```python
from build123d import *

# Parameters (mm, degrees)
SKETCH_W        = 196
SKETCH_H        = 200
PAD_DEPTH       = 3
SKETCH001_R     = 39.5
POCKET_DEPTH    = 5
SKETCH002_R     = 3.5
POCKET001_DEPTH = 5
SKETCH003_W     = 8
SKETCH003_H     = 180
PAD001_DEPTH    = 4
SKETCH004_W     = 160
SKETCH004_H     = 8
PAD002_DEPTH    = 4


with BuildPart() as part:
    # Sketch → Pad (new body)
    with BuildSketch(Plane.XY):
        Rectangle(SKETCH_W, SKETCH_H)
    extrude(amount=PAD_DEPTH)

    # Sketch001 (on Face6 of Pad) → Pocket (cut)
    with BuildSketch(Plane.XY.offset(3)):
        with Locations((-50, 50)):
            Circle(SKETCH001_R)
        with Locations((50, 50)):
            Circle(SKETCH001_R)
        with Locations((50, -50)):
            Circle(SKETCH001_R)
        with Locations((-50, -50)):
            Circle(SKETCH001_R)
    extrude(amount=-POCKET_DEPTH, mode=Mode.SUBTRACT)

    # Sketch002 (on Face5 of Pocket) → Pocket001 (cut)
    with BuildSketch(Plane.XY.offset(3)):
        with Locations((-91, 0)):
            Circle(SKETCH002_R)
        with Locations((88.593941, 0)):
            Circle(SKETCH002_R)
    extrude(amount=-POCKET001_DEPTH, mode=Mode.SUBTRACT)

    # Sketch003 (on Face5 of Pocket001) → Pad001 (join)
    with BuildSketch(Plane.XY.offset(3)):
        Rectangle(SKETCH003_W, SKETCH003_H)
    extrude(amount=PAD001_DEPTH)

    # Sketch004 (on Face5 of Pad001) → Pad002 (join)
    with BuildSketch(Plane.XY.offset(3)):
        Rectangle(SKETCH004_W, SKETCH004_H)
    extrude(amount=PAD002_DEPTH)


solid = part.part
```
CAD build for the part. Positions are in the model's coordinates, mm. Give positions to 0.01 mm unless a question says otherwise; leave off trailing zeros. Loops run counter-clockwise (first coordinate to the right, second up) from the corner with the lowest first, then second, coordinate; pieces in that order, holes last. Notation, with made-up numbers: (72, 79.5) - (101, 79.5) arc R11 ccw to (101, 89.5) - close; hole circle Ø4 at (75, 10). An arc over 180 degrees is marked (long way). Put each result on its own line as item: value.
Q1. Mould opens along Y. For faces 1 (the face through (68.23, -85.04, 1.52)), 2 (the face through (-1, 1, 0)) say: pulls with the +Y half, pulls with the -Y half, needs draft (parallel to the pull), parting line crosses it, or undercut.
Filled in:
face 1: undercut
face 2: needs draft
Q2. Slice it at C-C (z = 5.25). Give the cut face in (x, y).
Filled in:
outline: (-80, -4) - (-4, -4) - (-4, -90) - (4, -90) - (4, -4) - (80, -4) - (80, 4) - (4, 4) - (4, 90) - (-4, 90) - (-4, 4) - (-80, 4) - close
Q3. Probe line 1 along Y through (x, z) = (-50, 1.95); line 2 along X through (y, z) = (-24, 1.5); line 3 along Y through (x, z) = (-91, 1.45). List the from-to ranges inside material, lowest first.
Filled in:
line 1: y = -100 to -89.5, -10.5 to 10.5, 89.5 to 100
line 2: x = -98 to -79.74, -20.26 to 20.26, 79.74 to 98
line 3: y = -100 to -3.5, 3.5 to 100
Q4. Flat gauge pins, fed straight in: pin 1 (1.2 mm diameter, centred on y = 67.5, z = 6, fed in from -X); pin 2 (1.5 mm diameter, centred on x = 22, y = -76.5, fed in from +Z); pin 3 (1.2 mm diameter, centred on x = 40.5, z = 5.5, fed in from -Y); pin 4 (2 mm diameter, centred on y = -2, z = 4.5, fed in from +X). Where does each tip first touch, or does it go through?
Filled in:
pin 1: stops at x = -4
pin 2: passes through
pin 3: stops at y = -4
pin 4: stops at x = 80
Q5. Slice it at B-B (x = -50). Give the cut face in (y, z), plus the area to 3 significant figures.
Filled in:
outline: (-100, 0) - (-89.5, 0) - (-89.5, 3) - (-100, 3) - close; (-10.5, 0) - (10.5, 0) - (10.5, 3) - (4, 3) - (4, 7) - (-4, 7) - (-4, 3) - (-10.5, 3) - close; (89.5, 0) - (100, 0) - (100, 3) - (89.5, 3) - close
area: 158 mm²
Q6. Slice it at A-A (y = -50). Give the cut face in (x, z), plus the area to 3 significant figures.
Filled in:
outline: (-98, 0) - (-89.5, 0) - (-89.5, 3) - (-98, 3) - close; (-10.5, 0) - (10.5, 0) - (10.5, 3) - (4, 3) - (4, 7) - (-4, 7) - (-4, 3) - (-10.5, 3) - close; (89.5, 0) - (98, 0) - (98, 3) - (89.5, 3) - close
area: 146 mm²
